from build123d import *

# Parameters (mm, degrees)
SKETCH1_R           = 40
BOSS_EXTRUDE1_DEPTH = 240
SKETCH2_R           = 30
BOSS_EXTRUDE2_DEPTH = 15
SKETCH3_R           = 12.5
CUT_EXTRUDE2_DEPTH  = 10


with BuildPart() as part:
    # Sketch1 → Boss-Extrude1 (new body)
    with BuildSketch(Plane(origin=(0, 0, 0), x_dir=(1, 0, 0), z_dir=(0, 1, 0))):
        Circle(SKETCH1_R)
    extrude(amount=BOSS_EXTRUDE1_DEPTH)

    # Sketch2 → Boss-Extrude2 (add)
    with BuildSketch(Plane.XZ):
        Circle(SKETCH2_R)
    extrude(amount=BOSS_EXTRUDE2_DEPTH)

    # Sketch3 → Cut-Extrude2 (cut)
    with BuildSketch(Plane.XZ.offset(15)):
        Circle(SKETCH3_R)
    extrude(amount=-CUT_EXTRUDE2_DEPTH, mode=Mode.SUBTRACT)


solid = part.part
Can you work these out from the model? Positions are in its coordinate system, mm. A direction names the side the tool comes from. Coordinates: 2 decimals unless noted, no trailing zeros. Loops run counter-clockwise (first coordinate to the right, second up) from the corner with the lowest first, then second, coordinate; pieces in that order, holes last. Notation, with made-up numbers: M 88.25,-4 L 104.25,-4 A16 ccw 104.25,2 Z; hole C -25.5,64.25 d1. An arc over 180 degrees is marked long. Answer as CSV lines item,"result". Start each with the question number.
1. For pin 1 Ø8 at (x, y) = (-9, 198) entering from +Z; pin 2 Ø12 at (y, z) = (191.5, 30) entering from -X; pin 3 Ø12 at (y, z) = (163, -14.5) entering from +X, each with a flat end and sliding along its axis, tell me the tip position at first contact or that it passes through.
2. Thinking about a two-plate mould opening in Z: for faces 3 (the face through (11.923, -10.07, 3.755)), 4 (the face through (-8.67, 118.32, 39.05)), 5 (the face through (6, 0, -30)), which applies, +Z half, -Z half, draft (parallel to the pull), parting line (faces both ways), or undercut?
3. Suppose I cut it at B-B, the plane z = 0. List the corners of the cut face in (x, y) for me.
4. Suppose I cut it at D-D, the plane y = 112. List the corners of the cut face in (x, z) for me, plus the area to 3 significant figures.
5. If I drill on probe 1 along Z at (x, y) = (0, -8); probe 2 along Y at (x, z) = (-22, 31); probe 3 along Z at (x, y) = (-2, 127), over which ranges is the centre line in solid material (lowest first)? Write a range as [from, to].
6. Suppose I cut it at A-A, the plane x = -24. List the corners of the cut face in (y, z) for me.
7. Suppose I cut it at C-C, the plane x = 0. List the corners of the cut face in (y, z) for me.
8. For faces 1 (the face through (-29.97, -7.4, 1.32)), 2 (the face through (13, -15, 0)), which set-ups out of +Z, -Z, +X, -X, +Y, -Y let a thin tool reach every point of the face, with its end or its side?
Output:
1,pin 1,"stops at z = 39.69"
1,pin 2,"stops at x = -32"
1,pin 3,"stops at x = 39.09"
2,face 3,"undercut"
2,face 4,"parting line"
2,face 5,"draft"
3,outline,"M -40,0 L -30,0 L -30,-15 L -12.5,-15 L -12.5,-5 L 12.5,-5 L 12.5,-15 L 30,-15 L 30,0 L 40,0 L 40,240 L -40,240 Z"
4,outline,"C 0,0 d80"
4,area,"5,030 mm^2"
5,probe 1,"z = [-30, -12.5], [12.5, 30]"
5,probe 2,"y = [0, 240]"
5,probe 3,"z = [-39.95, 39.95]"
6,outline,"M -15,-18 L 0,-18 L 0,-32 L 240,-32 L 240,32 L 0,32 L 0,18 L -15,18 Z"
7,outline,"M -15,-30 L 0,-30 L 0,-40 L 240,-40 L 240,40 L 0,40 L 0,30 L -15,30 L -15,12.5 L -5,12.5 L -5,-12.5 L -15,-12.5 Z"
8,face 1,"-Y"
8,face 2,"+Z, -Z, +X, -X, -Y"
